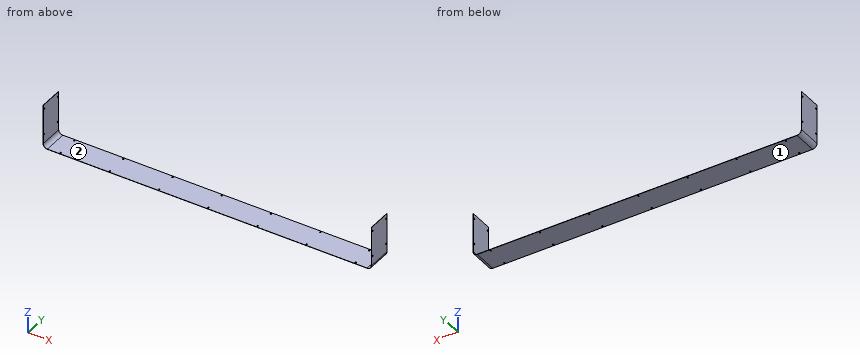
```python
from build123d import *

# Parameters (mm, degrees)
BASE_FLANGE1_DEPTH = 88
SKETCH2_R          = 2.5
CUT_EXTRUDE1_DEPTH = 1216.791100477
SKETCH3_R          = 2.5
CUT_EXTRUDE2_DEPTH = 10


# Read off the part's stored shape, not the designer's step: Base-Flange1
with BuildPart() as part:
    # Base-Flange1 outline → Base-Flange1 (new body)
    with BuildSketch(Plane(origin=(0, 0, 0), x_dir=(1, 0, 0), z_dir=(0, 1, 0))):
        with BuildLine():
            Line((1201, 144), (1201, 0))
            Line((1201, 0), (1202, 0))
            Line((1202, 0), (1202, 144))
            ThreePointArc((1202, 144), (1197.313708499, 155.313708499), (1186, 160))
            Line((1186, 160), (16, 160))
            ThreePointArc((16, 160), (4.686291501, 155.313708499), (0, 144))
            Line((0, 144), (0, 0))
            Line((0, 0), (1, 0))
            Line((1, 0), (1, 144))
            ThreePointArc((1, 144), (5.393398282, 154.606601718), (16, 159))
            Line((16, 159), (1186, 159))
            ThreePointArc((1186, 159), (1196.606601718, 154.606601718), (1201, 144))
        make_face()
    extrude(amount=BASE_FLANGE1_DEPTH)

    # Sketch2 → Cut-Extrude1 (cut, through all)
    with BuildSketch(Plane(origin=(1202, 0, 0), x_dir=(0, 0, -1), z_dir=(1, 0, 0))):
        with Locations((16, 82)):
            Circle(SKETCH2_R)
        with Locations((111, 82)):
            Circle(SKETCH2_R)
        with Locations(Location((111, 6, 0), (0, 0, 180))):
            Circle(SKETCH2_R)
        with Locations(Location((16, 6, 0), (0, 0, 180))):
            Circle(SKETCH2_R)
    extrude(amount=-CUT_EXTRUDE1_DEPTH, mode=Mode.SUBTRACT)

    # Sketch3 → Cut-Extrude2 (cut)
    with BuildSketch(Plane(origin=(0, 0, -160), x_dir=(-1, 0, 0), z_dir=(0, 0, -1))):
        with Locations((-1141, 82)):
            Circle(SKETCH3_R)
        with Locations((-961, 82)):
            Circle(SKETCH3_R)
        with Locations((-781, 82)):
            Circle(SKETCH3_R)
        with Locations((-601, 82)):
            Circle(SKETCH3_R)
        with Locations((-421, 82)):
            Circle(SKETCH3_R)
        with Locations((-241, 82)):
            Circle(SKETCH3_R)
        with Locations((-61, 82)):
            Circle(SKETCH3_R)
        with Locations((-961, 6)):
            Circle(SKETCH3_R)
        with Locations((-781, 6)):
            Circle(SKETCH3_R)
        with Locations((-601, 6)):
            Circle(SKETCH3_R)
        with Locations((-421, 6)):
            Circle(SKETCH3_R)
        with Locations((-241, 6)):
            Circle(SKETCH3_R)
        with Locations((-61, 6)):
            Circle(SKETCH3_R)
        with Locations((-1141, 6)):
            Circle(SKETCH3_R)
    extrude(amount=-CUT_EXTRUDE2_DEPTH, mode=Mode.SUBTRACT)


solid = part.part
```
Model file for the job. Use its own axes, mm. Face numbers are marked on the shaded views. Round coordinates to 2 decimals unless told otherwise and drop trailing zeros. Order: outer loops, then holes, each group sorted by start corner. A loop starts at its lowest first (then second) coordinate and runs counter-clockwise, first axis right, second up. Notation, with made-up numbers: M 61.25,15.5 L 70.25,15.5 A28 ccw 70.25,44.5 Z; hole C 17,-16.75 d8. An arc over 180 degrees is marked long. Use CSV: the item, a comma, the result in double quotes.
Item 1: Saw through at A-A (z = -43.5). List the corners of the cut face in (x, y), plus the area to 3 significant figures.
Worked answers:
outline,"M 0,0 L 1,0 L 1,88 L 0,88 Z; M 1201,0 L 1202,0 L 1202,88 L 1201,88 Z"
area,"176 mm²"
Item 2: Saw through at B-B (y = 46). List the corners of the cut face in (x, z).
Worked answers:
outline,"M 0,-144 A16 ccw 16,-160 L 1186,-160 A16 ccw 1202,-144 L 1202,0 L 1201,0 L 1201,-144 A15 cw 1186,-159 L 16,-159 A15 cw 1,-144 L 1,0 L 0,0 Z"
Item 3: Probe probe 1 along X at (y, z) = (67.5, -45.5); probe 2 along Z at (x, y) = (546, 60); probe 3 along X at (y, z) = (20, -149.5). List the from-to ranges inside material, lowest first.
Worked answers:
probe 1,"0 to 1, 1201 to 1202"
probe 2,"-160 to -159"
probe 3,"0.98 to 2.04, 1199.96 to 1201.02"
Item 4: Saw through at C-C (x = 293). List the corners of the cut face in (y, z), plus the area to 3 significant figures.
Worked answers:
outline,"M 0,-160 L 88,-160 L 88,-159 L 0,-159 Z"
area,"88.0 mm²"
Item 5: Pin check, flat tips, straight feed: pin 1 (3 mm diameter, centred on y = 82, z = -111, fed in from +X); pin 2 (3 mm diameter, centred on x = 707.5, y = 14.5, fed in from +Z); pin 3 (8 mm diameter, centred on x = 241, y = 82, fed in from -Z). Stop position of each tip, or through.
Worked answers:
pin 1,"through"
pin 2,"z = -159"
pin 3,"z = -160"
Item 6: Pull direction X, two halves, no side cores. Call the marked faces 1 and 2: released by +X, released by -X, zero draft, split by the parting line, or undercut.
Worked answers:
face 1,"zero draft"
face 2,"undercut"
